Check sheet for the drawn part. Datum: minimum x, y, z corner. Units: mm. A direction names the side the tool comes from. Give positions to 0.01 mm unless a question says otherwise; leave off trailing zeros. Order: outer loops, then holes, each group sorted by start corner. A loop starts at its lowest first (then second) coordinate and runs counter-clockwise, first axis right, second up. Notation, with made-up numbers: (-25.75, 62) -> (-11.75, 62) arc R22 ccw to (-11.75, 99) -> close; hole circle Ø8 at (-15.75, -22.75). An arc over 180 degrees is marked (long way). One line per question, with ' | ' between items. Start each with the question number.
Q1. Section check D-D on z = 33.5. Record the cut outline in (x, y), plus the area to 3 significant figures.
Q2. Section check B-B on x = 112. Record the cut outline in (y, z).
Q3. Material ranges on probe 1 along Y at (x, z) = (16, 8); probe 2 along Y at (x, z) = (67, 21); probe 3 along Z at (x, y) = (110.5, 105.5), recorded low to high. Write a range as [from, to].
Q4. Section check A-A on y = 111. Record the cut outline in (x, z).
Q5. Section check C-C on z = 9. Record the cut outline in (x, y), plus the area to 3 significant figures.
Q6. Access from +Z, -Z, +X, -X, +Y, -Y to the whole of each face (thin tool, end or side, straight path). Record for the marked faces 1, 2, 3 and 4.
Q7. Go/stop test with flat-tipped pins: pin 1 (12 mm diameter, centred on x = 29, z = 15.5, fed in from -Y); pin 2 (7.5 mm diameter, centred on y = 114.5, z = 58.5, fed in from +X); pin 3 (7.5 mm diameter, centred on x = 28, y = 112.5, fed in from +Z). Record where each tip stops, or that it passes through.
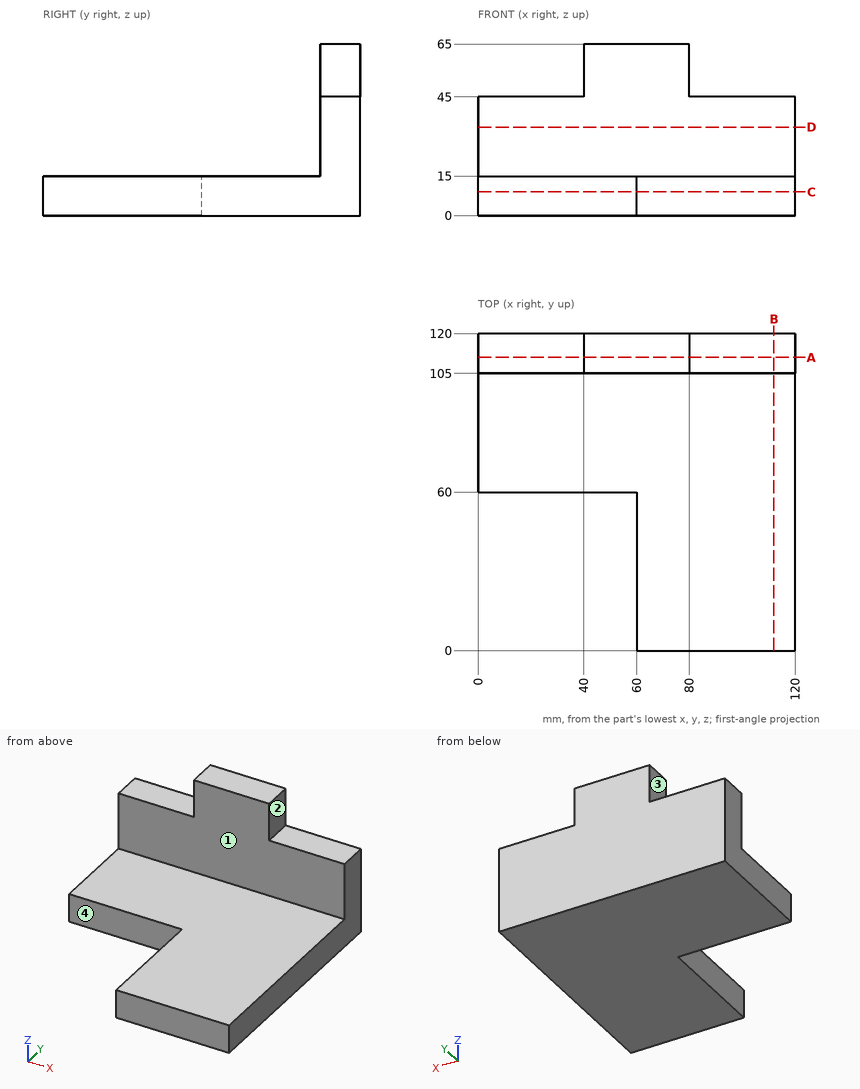
Filled in:
1) outline: (0, 105) -> (120, 105) -> (120, 120) -> (0, 120) -> close | area: 1,800 mm²
2) outline: (0, 0) -> (120, 0) -> (120, 45) -> (105, 45) -> (105, 15) -> (0, 15) -> close
3) probe 1: [60, 120] | probe 2: [105, 120] | probe 3: [0, 45]
4) outline: (0, 0) -> (120, 0) -> (120, 45) -> (80, 45) -> (80, 65) -> (40, 65) -> (40, 45) -> (0, 45) -> close
5) outline: (0, 60) -> (60, 60) -> (60, 0) -> (120, 0) -> (120, 120) -> (0, 120) -> close | area: 10,800 mm²
6) face 1: +Z, +X, -X, -Y | face 2: +Z, +X, +Y, -Y | face 3: +Z, -X, +Y, -Y | face 4: +Z, -Z, -X, -Y
7) pin 1: y = 60 | pin 2: x = 80 | pin 3: z = 45
